The listing builds one solid part. Answer for the finished solid, in the listing's coordinates (mm). A direction names the side the tool comes from. Give positions to 0.01 mm unless a question says otherwise; leave off trailing zeros. Write each loop counter-clockwise with the first axis right and the second up, starting at its lowest first coordinate (ties: lowest second). Pieces come first, ordered by that corner, then holes. Notation, with made-up numbers: (85.25, 72) -> (142.25, 72) arc R30 cw to (142.25, 110) -> close; hole circle Ø10 at (2, -3). An arc over 180 degrees is marked (long way). Put each result on its own line as item: value. Start each with the question number.
1) A cutting plane is placed at A-A (z = 22.5). Write down the section's boundary in (x, y) (3 decimals).
2) A cutting plane is placed at C-C (y = -7.5). Write down the section's boundary in (x, z) (3 decimals), then the cut area to 3 significant figures.
3) For a pull along Y with two mould halves and no side action, classify faces 6 (the cylindrical face through (-0.9, -24.78, 22.43)), 7 (the flat face through (40, -13, 3.175)), 8 (the cylindrical face through (82.41, -11.46, 0.92)) as released by +Y, released by -Y, zero draft, split by the parting line, or undercut.
4) Find the intervals of material crossed by line 1 along X through (y, z) = (-14.25, 37); line 2 along Y through (x, z) = (42.5, 35) (3 decimals); line 3 along Z through (x, y) = (69, -17.5) (3 decimals), in increasing order. Write a range as from..to.
5) A cutting plane is placed at D-D (z = 31.5). Write down the section's boundary in (x, y) (3 decimals), then the cut area to 3 significant figures.
6) Flat-ended cylindrical pins translate along their axes: pin 1 Ø3.5 at (x, y) = (88, -1) entering from -Z (3 decimals); pin 2 Ø6 at (y, z) = (-7.5, 17.5) entering from +X; pin 3 Ø14 at (x, z) = (-7.5, 33.5) entering from -Y. Find the tip coordinate at first contact, or state that the pin passes through.
7) A cutting plane is placed at B-B (x = 24). Write down the section's boundary in (y, z) (3 decimals), then the cut area to 3 significant figures.
8) For faces 1 (the flat face through (95.976, -2, 35)), 2 (the flat face through (88, -3.175, 36)), 3 (the flat face through (90, -2, 28.575)), 4 (the flat face through (40, -22.479, 22)), 5 (the cylindrical face through (91.15, -1.57, 34.99)), determine the directions among +Z, -Z, +X, -X, +Y, -Y from which every point of the face is accessible in a straight line to the end or side of a thin tool.
from build123d import *

# Parameters (mm, degrees)
F0_W     = 85.09
F0_H     = 41.275
F1_DEPTH = 25.654
F2_T     = -3.175
F3_W     = 12.7
F3_H     = 12.7
F3_R     = 1.524
F4_DEPTH = 3.175
F5_R     = 3.048


with BuildPart() as f1:
    # F0 (on Front) → F1 (new body)
    with BuildSketch(Plane.XZ):
        with Locations((40.730714, 20.6375)):
            Rectangle(F0_W, F0_H)
    extrude(amount=F1_DEPTH)

    # F2
    f2_openings = [f1.faces().sort_by_distance(p)[0] for p in [
        (40.730714, -12.827, 41.275),
    ]]
    offset(amount=F2_T, openings=f2_openings)

    # F3 (on face) → F4 (join)
    with BuildSketch(Plane(origin=(0, 0, 0), x_dir=(-1, 0, 0), z_dir=(0, 1, 0))):
        with Locations((8.164286, 34.925)):
            Rectangle(F3_W, F3_H)
        with Locations((8.164286, 34.925)):
            Circle(F3_R, mode=Mode.SUBTRACT)
        with Locations((-89.625714, 34.925)):
            Rectangle(F3_W, F3_H)
        with Locations((-89.625714, 34.925)):
            Circle(F3_R, mode=Mode.SUBTRACT)
    extrude(amount=-F4_DEPTH)

    # F5
    f5_edges = [f1.edges().sort_by_distance(p)[0] for p in [
        (40.730714, -25.654, 41.275),
        (-1.814286, -25.654, 20.6375),
        (40.730714, -25.654, 0),
        (83.275714, -25.654, 20.6375),
        (83.275714, -12.827, 0),
        (-1.814286, -12.827, 0),
    ]]
    fillet(f5_edges, radius=F5_R)


solid = f1.part
Reply:
1. outline: (-1.814, -22.606) arc R3.048 ccw to (1.234, -25.654) -> (80.228, -25.654) arc R3.048 ccw to (83.276, -22.606) -> (83.276, 0) -> (-1.814, 0) -> close; hole (1.361, -22.479) -> (80.101, -22.479) -> (80.101, -3.175) -> (1.361, -3.175) -> close
2. outline: (-1.814, 3.048) arc R3.048 ccw to (1.234, 0) -> (80.228, 0) arc R3.048 ccw to (83.276, 3.048) -> (83.276, 41.275) -> (80.101, 41.275) -> (80.101, 3.175) -> (1.361, 3.175) -> (1.361, 41.275) -> (-1.814, 41.275) -> close
2. area: 508 mm2
3. face 6: released by -Y
3. face 7: undercut
3. face 8: zero draft
4. line 1: x = -1.81..1.36, 80.1..83.28
4. line 2: y = -25.654..-22.479, -3.175..0
4. line 3: z = 0..3.175
5. outline: (-14.514, -3.175) -> (-1.814, -3.175) -> (-1.814, -22.606) arc R3.048 ccw to (1.234, -25.654) -> (80.228, -25.654) arc R3.048 ccw to (83.276, -22.606) -> (83.276, -3.175) -> (95.976, -3.175) -> (95.976, 0) -> (-14.514, 0) -> close; hole (1.361, -22.479) -> (80.101, -22.479) -> (80.101, -3.175) -> (1.361, -3.175) -> close
5. area: 740 mm2
6. pin 1: stops at z = 28.575
6. pin 2: stops at x = 83.28
6. pin 3: stops at y = -25.11
7. outline: (-25.654, 3.048) arc R3.048 ccw to (-22.606, 0) -> (0, 0) -> (0, 41.275) -> (-3.175, 41.275) -> (-3.175, 3.175) -> (-22.479, 3.175) -> (-22.479, 41.275) -> (-22.606, 41.275) arc R3.048 ccw to (-25.654, 38.227) -> close
7. area: 319 mm2
8. face 1: +Z, -Z, +X, +Y, -Y
8. face 2: +Z, -Z, +X, -Y
8. face 3: -Z, +X, +Y, -Y
8. face 4: +Z
8. face 5: +Y, -Y
